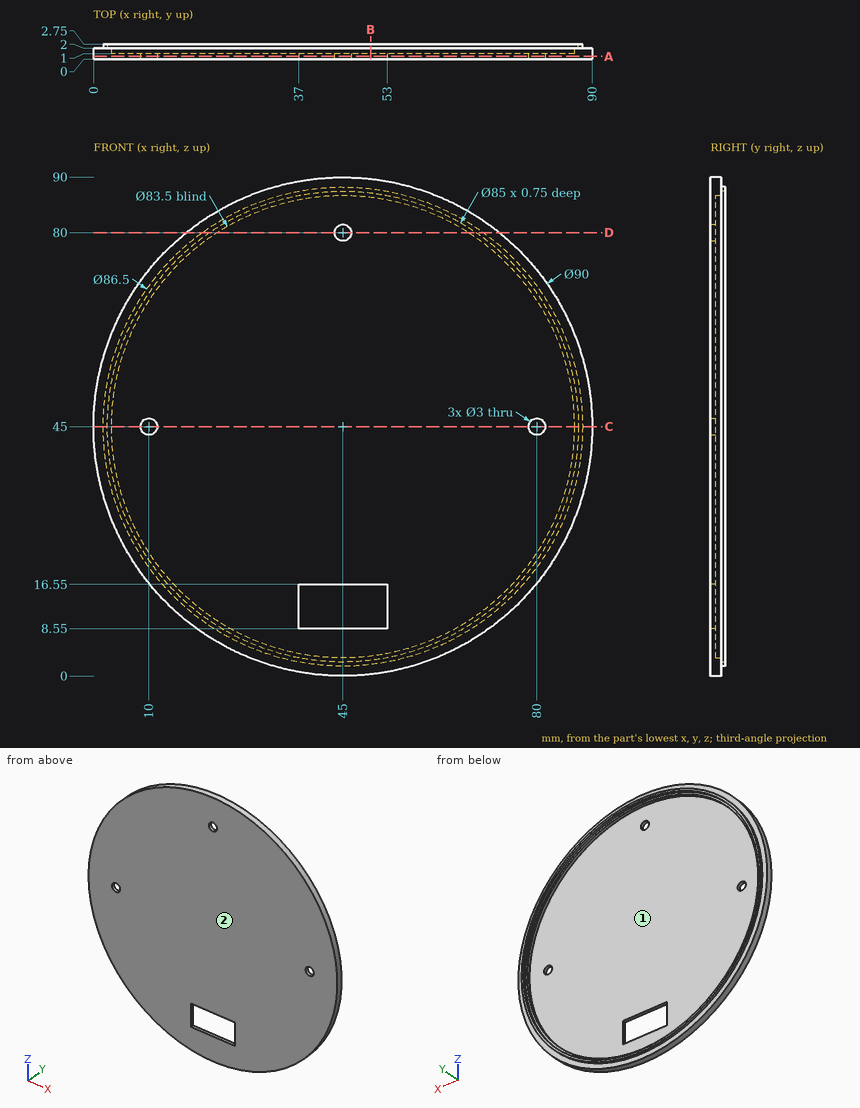
Print and shaded views of the part. All mm, measured from the part's lowest x, y and z. Round coordinates to 2 decimals unless told otherwise and drop trailing zeros. Write each loop counter-clockwise with the first axis right and the second up, starting at its lowest first coordinate (ties: lowest second). Pieces come first, ordered by that corner, then holes. Notation, with made-up numbers: (62.25, -5) - (119.25, -5) arc R14 ccw to (119.25, 13) - close; hole circle Ø11 at (88, 73). An arc over 180 degrees is marked (long way). One line per item, written item: value.
(1) Two-plate mould, pull along X, no slides. Class the marked faces 1 and 2: pulls with the +X half, pulls with the -X half, needs draft (parallel to the pull), parting line crosses it, or undercut.
Values follow:
face 1: undercut
face 2: needs draft
(2) Cut at B-B, the plane x = 50. Give the cut face in (y, z).
Values follow:
outline: (0, 0.28) - (2, 0.28) - (2, 2.04) - (2.75, 2.04) - (2.75, 2.8) - (2, 2.8) - (2, 3.55) - (1, 3.55) - (1, 8.55) - (0, 8.55) - close; (0, 16.55) - (1, 16.55) - (1, 86.45) - (2, 86.45) - (2, 87.2) - (2.75, 87.2) - (2.75, 87.96) - (2, 87.96) - (2, 89.72) - (0, 89.72) - close
(3) Wall check: probe 1 along X at (y, z) = (2.55, 45); probe 2 along Z at (x, y) = (45, 1.6); probe 3 along X at (y, z) = (2.3, 37.5). Give the ranges that are in metal, low to high.
Values follow:
probe 1: x = 1.75 to 2.5, 87.5 to 88.25
probe 2: z = 0 to 3.25, 86.75 to 90
probe 3: x = 2.41 to 3.17, 86.83 to 87.59
(4) Drop flat-ended pins along their axis: P1, Ø1.5, axis at x = 52.5, z = 33, coming from the -Y side; P2, Ø4, axis at x = 10, z = 45, coming from the +Y side; P3, Ø0.8, axis at x = 42, y = 0.5, coming from the -Z side; P4, Ø0.5, axis at y = 0.5, z = 14, coming from the -X side. Give the stop position or say it passes through.
Values follow:
P1: stops at y = 0
P2: stops at y = 1
P3: stops at z = 0.08
P4: stops at x = 12.15
(5) Cut at D-D, the plane z = 80. Give the cut face in (x, y), plus the area to 3 significant figures.
Values follow:
outline: (16.72, 0) - (43.5, 0) - (43.5, 1) - (22.24, 1) - (22.24, 2) - (20.89, 2) - (20.89, 2.75) - (19.59, 2.75) - (19.59, 2) - (16.72, 2) - close; (46.5, 0) - (73.28, 0) - (73.28, 2) - (70.41, 2) - (70.41, 2.75) - (69.11, 2.75) - (69.11, 2) - (67.76, 2) - (67.76, 1) - (46.5, 1) - close
area: 66.6 mm²
(6) Cut at C-C, the plane z = 45. Give the cut face in (x, y).
Values follow:
outline: (0, 0) - (8.5, 0) - (8.5, 1) - (3.25, 1) - (3.25, 2) - (2.5, 2) - (2.5, 2.75) - (1.75, 2.75) - (1.75, 2) - (0, 2) - close; (11.5, 0) - (78.5, 0) - (78.5, 1) - (11.5, 1) - close; (81.5, 0) - (90, 0) - (90, 2) - (88.25, 2) - (88.25, 2.75) - (87.5, 2.75) - (87.5, 2) - (86.75, 2) - (86.75, 1) - (81.5, 1) - close
(7) Cut at A-A, the plane y = 0.5. Give the cut face in (x, z).
Values follow:
outline: circle Ø90 at (45, 45); hole circle Ø3 at (10, 45); hole (37, 8.55) - (53, 8.55) - (53, 16.55) - (37, 16.55) - close; hole circle Ø3 at (45, 80); hole circle Ø3 at (80, 45)
